Geometry check sheet. Reference: the model listing, model coordinates, mm. Round coordinates to 2 decimals unless told otherwise and drop trailing zeros. Write each loop counter-clockwise with the first axis right and the second up, starting at its lowest first coordinate (ties: lowest second). Pieces come first, ordered by that corner, then holes. Notation, with made-up numbers: (-11, 73) -> (33, 73) arc R24 cw to (33, 93) -> close; hole circle Ø1 at (25, 74). An arc over 180 degrees is marked (long way). Put each result on its own line as item: value. Start each with the question number.
Autodesk Inventor part; units mm, degrees
ref_plane "YZ Plane" through (0, 0, 0) normal (1, 0, 0) x (0, 1, 0)
ref_plane "XZ Plane" through (0, 0, 0) normal (0, 1, 0) x (-1, 0, 0)
ref_plane "XY Plane" through (0, 0, 0) normal (0, 0, 1) x (1, 0, 0)
sketch "Эскиз1" plane through (0, 0, 0) normal (0, 1, 0) x (-1, 0, 0)
  circle A0 centre (169.2619, 20) radius 1.1
  line L0 (100.131, 30.85) -> (105.631, 30.85)
  line L1 (105.631, 30.85) -> (105.631, 9.15)
  line L2 (105.631, 9.15) -> (100.131, 9.15)
  line L3 (100.131, 9.15) -> (100.131, 30.85)
  arc A1 (0, 40) -> (-0.5, 39.5) centre (0, 39.5) ccw
  line L4 (-0.5, 0.5) -> (-0.5, 39.5)
  arc A2 (-0.5, 0.5) -> (0, 0) centre (0, 0.5) ccw
  line L5 (172.2619, 0) -> (0, 0)
  arc A3 (172.2619, 0) -> (172.7619, 0.5) centre (172.2619, 0.5) ccw
  line L6 (172.7619, 39.5) -> (172.7619, 0.5)
  arc A4 (172.7619, 39.5) -> (172.2619, 40) centre (172.2619, 39.5) ccw
  line L7 (0, 40) -> (172.2619, 40)
  circle A5 centre (3, 20) radius 1.1
extrude "Выдавливание1" add sketch "Эскиз1" along normal blind 0.5
properties part number "metal_cap_forPrint"
(1) Sectioned sample at A-A (z = 24). Record the cut outline in (x, y).
(2) Go/stop test with a flat-tipped pin: pin 1 Ø2 at (x, z) = (-3, 20) entering from -Y. Record where the tip stops, or that it passes through.
(3) Material ranges on L1, parallel to X at y = 0.15, z = 13; L2, parallel to Z at x = -3, y = 0.4; L3, parallel to X at y = 0.1, z = 19, recorded low to high. Write a range as from..to.
(4) Sectioned sample at B-B (y = 0.1). Record the cut outline in (x, z).
Found:
1. outline: (-172.76, 0) -> (-105.63, 0) -> (-105.63, 0.5) -> (-172.76, 0.5) -> close; (-100.13, 0) -> (0.5, 0) -> (0.5, 0.5) -> (-100.13, 0.5) -> close
2. pin 1: through
3. L1: -172.76..-105.63, -100.13..0.5
3. L2: 0..18.9, 21.1..40
3. L3: -172.76..-169.72, -168.8..-105.63, -100.13..-3.46, -2.54..0.5
4. outline: (-172.76, 0.5) arc R0.5 ccw to (-172.26, 0) -> (0, 0) arc R0.5 ccw to (0.5, 0.5) -> (0.5, 39.5) arc R0.5 ccw to (0, 40) -> (-172.26, 40) arc R0.5 ccw to (-172.76, 39.5) -> close; hole circle Ø2.2 at (-169.26, 20); hole (-105.63, 9.15) -> (-100.13, 9.15) -> (-100.13, 30.85) -> (-105.63, 30.85) -> close; hole circle Ø2.2 at (-3, 20)
